Design review of the part built by this model. Coordinates are the model's own, in mm. A direction names the side the tool comes from. Coordinates: 2 decimals unless noted, no trailing zeros. Write each loop counter-clockwise with the first axis right and the second up, starting at its lowest first coordinate (ties: lowest second). Pieces come first, ordered by that corner, then holes.
Q1. The part is to be moulded in two halves that separate along X. For faces 1 (the flat face through (-25.4, 0, 1)), 2 (the flat face through (0, -12, -45.974)), 3 (the cylindrical face through (5.397, 11.917, 7.125)), say which applies: released by +X, released by -X, zero draft, split by the parting line, or undercut.
Q2. For pin 1 Ø4 at (x, z) = (6.35, 4.826) entering from -Y, flat-tipped, find the tip position at first contact; note if it passes through.
Q3. Take a section at B-B, the plane z = -29.5. Write out the cut boundary in (x, y).
Q4. For faces 4 (the flat face through (23.812, 0, 1)), 5 (the flat face through (0, 12.7, 1)), list the 3-axis set-ups (+Z, -Z, +X, -X, +Y, -Y) from which the entire face can be reached by the end or side of a thin tool; tool diameter is ignored.
Q5. Take a section at C-C, the plane y = 5.25. Write out the cut boundary in (x, z).
Q6. For L1, parallel to Y at x = -11, z = 19; L2, parallel to X at y = -8, z = 29, list the stretches that pass through material, from the lowest coordinate up.
Q7. Take a section at A-A, the plane x = 6.35. Write out the cut boundary in (y, z).
Q8. Take a section at D-D, the plane x = 18. Write out the cut boundary in (y, z), plus the area to 3 significant figures.
from build123d import *

# Parameters (mm, degrees)
SKETCH1_W           = 50.8
SKETCH1_H           = 25.4
SKETCH1_W_2         = 47.625
SKETCH1_H_2         = 22.225
BOSS_EXTRUDE1_DEPTH = 45.974
SKETCH2_R           = 2.4892
CUT_EXTRUDE1_DEPTH  = 59.343197341


with BuildPart() as part:
    # Sketch1 → Boss-Extrude1 (new, symmetric)
    with BuildSketch(Plane.XY):
        Rectangle(SKETCH1_W, SKETCH1_H)
        Rectangle(SKETCH1_W_2, SKETCH1_H_2, mode=Mode.SUBTRACT)
    extrude(amount=BOSS_EXTRUDE1_DEPTH, both=True)

    # Sketch2 → Cut-Extrude1 (cut, through all)
    with BuildSketch(Plane(origin=(0, 12.7, 0), x_dir=(1, 0, 0), z_dir=(0, 1, 0))):
        with Locations(Location((-6.35, -4.826, 0), (0, 0, 270))):
            Circle(SKETCH2_R)
        with Locations(Location((6.35, -4.826, 0), (0, 0, 270))):
            Circle(SKETCH2_R)
        with Locations(Location((-6.35, -17.526, 0), (0, 0, 270))):
            Circle(SKETCH2_R)
        with Locations(Location((6.35, -17.526, 0), (0, 0, 270))):
            Circle(SKETCH2_R)
    extrude(amount=-CUT_EXTRUDE1_DEPTH, mode=Mode.SUBTRACT)


solid = part.part
Responses:
1. face 1: released by -X
1. face 2: zero draft
1. face 3: undercut
2. pin 1: passes through
3. outline: (-25.4, -12.7) - (25.4, -12.7) - (25.4, 12.7) - (-25.4, 12.7) - close; hole (-23.81, -11.11) - (23.81, -11.11) - (23.81, 11.11) - (-23.81, 11.11) - close
4. face 4: +Z, -Z
4. face 5: +Z, -Z, +X, -X, +Y
5. outline: (-25.4, -45.97) - (-23.81, -45.97) - (-23.81, 45.97) - (-25.4, 45.97) - close; (23.81, -45.97) - (25.4, -45.97) - (25.4, 45.97) - (23.81, 45.97) - close
6. L1: y = -12.7 to -11.11, 11.11 to 12.7
6. L2: x = -25.4 to -23.81, 23.81 to 25.4
7. outline: (-12.7, -45.97) - (-11.11, -45.97) - (-11.11, 2.34) - (-12.7, 2.34) - close; (-12.7, 7.32) - (-11.11, 7.32) - (-11.11, 15.04) - (-12.7, 15.04) - close; (-12.7, 20.02) - (-11.11, 20.02) - (-11.11, 45.97) - (-12.7, 45.97) - close; (11.11, -45.97) - (12.7, -45.97) - (12.7, 2.34) - (11.11, 2.34) - close; (11.11, 7.32) - (12.7, 7.32) - (12.7, 15.04) - (11.11, 15.04) - close; (11.11, 20.02) - (12.7, 20.02) - (12.7, 45.97) - (11.11, 45.97) - close
8. outline: (-12.7, -45.97) - (-11.11, -45.97) - (-11.11, 45.97) - (-12.7, 45.97) - close; (11.11, -45.97) - (12.7, -45.97) - (12.7, 45.97) - (11.11, 45.97) - close
8. area: 292 mm2
